Build history of the part. All positions in model axes, mm. A direction names the side the tool comes from. Give positions to 0.01 mm unless a question says otherwise; leave off trailing zeros. Loops run counter-clockwise (first coordinate to the right, second up) from the corner with the lowest first, then second, coordinate; pieces in that order, holes last. Notation, with made-up numbers: (56, 28) -> (84, 28) arc R31 ccw to (84, 58) -> close; hole circle Ø5 at (-16, -29.5). An arc over 180 degrees is marked (long way). One line per question, with ' | ' between items. Start each with the question number.
(1) 3-axis set-ups, long thin cutter, end or side, ignore diameter. For faces 4 (the face through (0, -25, 0)), 5 (the face through (0, -20, 0)), 6 (the face through (13, -7, 0)): which of +Z, -Z, +X, -X, +Y, -Y reach the whole face in a straight line?
(2) Slice it at A-A, the plane x = 0. Write the cut outline in (y, z), then the cut area to 3 significant figures.
(3) Mould opens along X. For faces 1 (the face through (11.923, -15.874, 3.755)), 2 (the face through (21.31, -3.45, -1)), 3 (the face through (6, 0, 0)) say: pulls with the +X half, pulls with the -X half, needs draft (parallel to the pull), parting line crosses it, or undercut.
(4) Slice it at C-C, the plane y = -1.75. Write the cut outline in (x, z).
(5) Drill centre lines: L1, parallel to Z at x = 0, y = -5; L2, parallel to Z at x = 0, y = -10.5; L3, parallel to Y at x = -18, z = 13.5. Where is each one in solid material? Low to high. Write a range as from..to.
(6) Flat gauge pins, fed straight in: pin 1 Ø4.5 at (x, z) = (20, 0) entering from -Y; pin 2 Ø1 at (x, y) = (8, -18) entering from +Z; pin 3 Ø8 at (x, y) = (-2.5, -16) entering from +Z; pin 4 Ø9 at (x, z) = (1.5, 1.5) entering from +Y. Where does each tip first touch, or does it go through?
(7) Slice it at D-D, the plane z = 20. Write the cut outline in (x, y).
(8) Slice it at B-B, the plane z = 0. Write the cut outline in (x, y).
```python
from build123d import *

# Parameters (mm, degrees)
F0_R     = 30
F1_DEPTH = 7
F3_D     = 3.3
F4_R     = 12.5
F5_DEPTH = 18
F6_R     = 4
F7_DEPTH = 20
F8_R     = 42.262069542
F9_DEPTH = 25


with BuildPart() as f1:
    # F0 (on Front) → F1 (new body)
    with BuildSketch(Plane.XZ):
        Circle(F0_R)
    extrude(amount=F1_DEPTH)

    # F3 (through all)
    with Locations(Plane.XZ.offset(7)):
        with Locations((0, 20), (20, 0), (0, -20), (-20, 0)):
            Hole(F3_D / 2)

    # F4 (on face) → F5 (join)
    with BuildSketch(Plane.XZ.offset(7)):
        Circle(F4_R)
    extrude(amount=F5_DEPTH)

    # F6 (on face) → F7 (cut)
    with BuildSketch(Plane(origin=(0, 0, 0), x_dir=(-1, 0, 0), z_dir=(0, 1, 0))):
        Circle(F6_R)
    extrude(amount=-F7_DEPTH, mode=Mode.SUBTRACT)


with BuildPart() as f9:
    # F8 (on Front) → F9 (new body)
    with BuildSketch(Plane.XZ):
        Circle(F8_R)
    extrude(amount=F9_DEPTH)


solid = f1.part
```
Final values:
1) face 4: +Z, -Z, +X, -X, -Y | face 5: +Y | face 6: -Y
2) outline: (-25, -12.5) -> (-7, -12.5) -> (-7, -18.35) -> (0, -18.35) -> (0, -4) -> (-20, -4) -> (-20, 4) -> (0, 4) -> (0, 18.35) -> (-7, 18.35) -> (-7, 12.5) -> (-25, 12.5) -> close; (-7, -30) -> (0, -30) -> (0, -21.65) -> (-7, -21.65) -> close; (-7, 21.65) -> (0, 21.65) -> (0, 30) -> (-7, 30) -> close | area: 664 mm2
3) face 1: parting line crosses it | face 2: undercut | face 3: needs draft
4) outline: circle Ø60 at (0, 0); hole circle Ø3.3 at (-20, 0); hole circle Ø8 at (0, 0); hole circle Ø3.3 at (0, -20); hole circle Ø3.3 at (0, 20); hole circle Ø3.3 at (20, 0)
5) L1: -30..-21.65, -18.35..-4, 4..18.35, 21.65..30 | L2: -12.5..-4, 4..12.5 | L3: -7..0
6) pin 1: y = -7 | pin 2: z = 10 | pin 3: z = 12.5 | pin 4: y = 0
7) outline: (-22.36, -7) -> (-1.65, -7) -> (-1.65, 0) -> (-22.36, 0) -> close; (1.65, -7) -> (22.36, -7) -> (22.36, 0) -> (1.65, 0) -> close
8) outline: (-30, -7) -> (-21.65, -7) -> (-21.65, 0) -> (-30, 0) -> close; (-18.35, -7) -> (-12.5, -7) -> (-12.5, -25) -> (12.5, -25) -> (12.5, -7) -> (18.35, -7) -> (18.35, 0) -> (4, 0) -> (4, -20) -> (-4, -20) -> (-4, 0) -> (-18.35, 0) -> close; (21.65, -7) -> (30, -7) -> (30, 0) -> (21.65, 0) -> close
